from build123d import *

# Parameters (mm, degrees)
F0_W     = 66.5
F0_H     = 80.5
F1_DEPTH = 12
F2_T     = -2.5
F3_R     = 2


with BuildPart() as f1:
    # F0 (on Front) → F1 (new body)
    with BuildSketch(Plane.XZ):
        with Locations((30.75, 37.75)):
            Rectangle(F0_W, F0_H)
    extrude(amount=F1_DEPTH)

    # F2
    f2_openings = [f1.faces().sort_by_distance(p)[0] for p in [
        (30.75, -12, 37.75),
    ]]
    offset(amount=F2_T, openings=f2_openings)

    # F3
    f3_edges = [f1.edges().sort_by_distance(p)[0] for p in [
        (64, -6, 78),
        (-2.5, -6, 78),
        (64, -6, -2.5),
        (-2.5, -6, -2.5),
    ]]
    fillet(f3_edges, radius=F3_R)


solid = f1.part
Design review of the part built by this model. Coordinates are the model's own, in mm. A direction names the side the tool comes from. Round coordinates to 2 decimals unless told otherwise and drop trailing zeros. Loops run counter-clockwise (first coordinate to the right, second up) from the corner with the lowest first, then second, coordinate; pieces in that order, holes last. Notation, with made-up numbers: (29, -16) - (63, -16) arc R24 ccw to (63, -3) - close; hole circle Ø2 at (-29, 43). An arc over 180 degrees is marked (long way). One line per question, with ' | ' between items.
1. Clearance check with flat-ended pins moving along their axes: P1, Ø8, axis at x = 33.5, z = 19.5, coming from the +Y side; P2, Ø3, axis at x = 46, z = 68.5, coming from the -Y side. State where each tip first meets the part, or that it passes through.
Results are:
P1: stops at y = 0 | P2: stops at y = -2.5
2. For faces 1 (the face through (63.4, -6.08, -1.93)), 2 (the face through (30, -7, 0)), list the 3-axis set-ups (+Z, -Z, +X, -X, +Y, -Y) from which the entire face can be reached by the end or side of a thin tool; tool diameter is ignored.
Results are:
face 1: -Z, +X, +Y, -Y | face 2: -Y
3. We need section C-C, the plane z = 72. State the section outline as (x, y) points, and give its area (3 significant figures).
Results are:
outline: (-2.5, -12) - (0, -12) - (0, -2.5) - (61.5, -2.5) - (61.5, -12) - (64, -12) - (64, 0) - (-2.5, 0) - close | area: 214 mm²
4. We need section A-A, the plane x = 3. State the section outline as (y, z) points, and give its area (3 significant figures).
Results are:
outline: (-12, -2.5) - (0, -2.5) - (0, 78) - (-12, 78) - (-12, 75.5) - (-2.5, 75.5) - (-2.5, 0) - (-12, 0) - close | area: 249 mm²
5. For L1, parallel to X at y = -3.5, z = 48.5; L2, parallel to Z at x = 8, y = -9.5; L3, parallel to Y at x = 37, z = 12, list the stretches that pass through material, from the lowest coordinate up. Write a range as [from, to].
Results are:
L1: x = [-2.5, 0], [61.5, 64] | L2: z = [-2.5, 0], [75.5, 78] | L3: y = [-2.5, 0]
6. We need section B-B, the plane y = -11. State the section outline as (x, z) points.
Results are:
outline: (-2.5, -0.5) arc R2 ccw to (-0.5, -2.5) - (62, -2.5) arc R2 ccw to (64, -0.5) - (64, 76) arc R2 ccw to (62, 78) - (-0.5, 78) arc R2 ccw to (-2.5, 76) - close; hole (0, 0) - (61.5, 0) - (61.5, 75.5) - (0, 75.5) - close
7. Draft analysis for pull direction X (two halves, no side actions). For faces 3 (the face through (-1.93, -6.08, 77.4)), 4 (the face through (30, -2.5, 38)), 5 (the face through (30, -6, -2.5)), state which applies: released by +X, released by -X, zero draft, split by the parting line, or undercut.
Results are:
face 3: released by -X | face 4: undercut | face 5: zero draft
